Can you work these out from the model? Positions are in its coordinate system, mm. A direction names the side the tool comes from. Coordinates: 2 decimals unless noted, no trailing zeros. Loops run counter-clockwise (first coordinate to the right, second up) from the corner with the lowest first, then second, coordinate; pieces in that order, holes last.
```python
from build123d import *

# Parameters (mm, degrees)
SKETCH001_R                          = 4
SKETCH001_R_2                        = 1.4
SKETCH001_R_3                        = 2.75
EXTRUDE001_DEPTH                     = 20
SKETCH002_AS_DRAWN_W                 = 15
SKETCH002_AS_DRAWN_H                 = 13
SKETCH002_AS_DRAWN_R                 = 3.35
EXTRUDE002_DEPTH                     = 3
EXTRUDE002_ONTO_SKETCH002_ROLL_ANGLE = 90
SKETCH_R                             = 1.9
SKETCH_R_2                           = 23
SKETCH_R_3                           = 1.85
EXTRUDE_DEPTH                        = 3
CHAMFER_SIZE                         = 0.6


with BuildPart() as extrude001:
    # Sketch001 → Extrude001 (new body)
    with BuildSketch(Plane.XY):
        with Locations((-50.25, -47.25)):
            Circle(SKETCH001_R)
        with Locations((-50.25, -47.25)):
            Circle(SKETCH001_R_2, mode=Mode.SUBTRACT)
        with Locations((50.25, 47.25)):
            Circle(SKETCH001_R)
        with Locations((50.25, 47.25)):
            Circle(SKETCH001_R_2, mode=Mode.SUBTRACT)
        with Locations((-50.25, 47.25)):
            Circle(SKETCH001_R)
        with Locations((-50.25, 47.25)):
            Circle(SKETCH001_R_2, mode=Mode.SUBTRACT)
        with Locations((25.25, -42.25)):
            Circle(SKETCH001_R)
        with Locations((25.25, -42.25)):
            Circle(SKETCH001_R_2, mode=Mode.SUBTRACT)
        with Locations((51.25, -51.75)):
            Circle(SKETCH001_R_3)
        with Locations((-14.75, -39.25)):
            Circle(SKETCH001_R)
        with Locations((-14.75, -39.25)):
            Circle(SKETCH001_R_2, mode=Mode.SUBTRACT)
    extrude(amount=EXTRUDE001_DEPTH)


with BuildPart() as extrude002:
    # Sketch002 as drawn → Extrude002 (new)
    with BuildSketch(Plane.XY):
        with Locations((0, 6.5)):
            Rectangle(SKETCH002_AS_DRAWN_W, SKETCH002_AS_DRAWN_H)
        with Locations((0, 7)):
            Circle(SKETCH002_AS_DRAWN_R, mode=Mode.SUBTRACT)
    extrude(amount=-EXTRUDE002_DEPTH)


with BuildPart() as extrude002_1:
    # Extrude002 onto Sketch002 roll: moved
    add(extrude002.part.rotate(Axis((0, 0, 0), (1, 0, 0)), EXTRUDE002_ONTO_SKETCH002_ROLL_ANGLE))


with BuildPart() as extrude002_2:
    # Extrude002 onto Sketch002 placement: moved
    add(extrude002_1.part)


with BuildPart() as extrude002_3:
    # Extrude002 placement: moved
    add(extrude002_2.part.moved(Location((32, 61, 2))))


with BuildPart() as chamfer_body:
    # Sketch → Extrude (new body)
    with BuildSketch(Plane.XY):
        Polygon((55.5, 55), (55.5, -55), (-55.5, -55), (-55.5, 55), (24.5, 55), (24.5, 65), (39.5, 65), (39.5, 55), align=None)
        with Locations((-50.25, -47.25)):
            Circle(SKETCH_R, mode=Mode.SUBTRACT)
        Circle(SKETCH_R_2, mode=Mode.SUBTRACT)
        with Locations((-39.25, 47.25)):
            Circle(SKETCH_R_3, mode=Mode.SUBTRACT)
        with Locations((0.75, 47.25)):
            Circle(SKETCH_R_3, mode=Mode.SUBTRACT)
        with Locations((-39.25, 32.25)):
            Circle(SKETCH_R_3, mode=Mode.SUBTRACT)
        with Locations((0.75, 32.25)):
            Circle(SKETCH_R_3, mode=Mode.SUBTRACT)
        with Locations((10.75, 44.25)):
            Circle(SKETCH_R_3, mode=Mode.SUBTRACT)
        with Locations((40.75, 44.25)):
            Circle(SKETCH_R_3, mode=Mode.SUBTRACT)
        with Locations((10.75, 32.25)):
            Circle(SKETCH_R_3, mode=Mode.SUBTRACT)
        with Locations((40.75, 32.25)):
            Circle(SKETCH_R_3, mode=Mode.SUBTRACT)
        with Locations((50.25, 47.25)):
            Circle(SKETCH_R, mode=Mode.SUBTRACT)
        with Locations((-50.25, 47.25)):
            Circle(SKETCH_R, mode=Mode.SUBTRACT)
        with Locations((25.25, -42.25)):
            Circle(SKETCH_R, mode=Mode.SUBTRACT)
        with Locations((-14.75, -39.25)):
            Circle(SKETCH_R, mode=Mode.SUBTRACT)
        with Locations((-37.25, -7.25)):
            Circle(SKETCH_R_3, mode=Mode.SUBTRACT)
        with Locations((-37.25, -47.25)):
            Circle(SKETCH_R_3, mode=Mode.SUBTRACT)
    extrude(amount=EXTRUDE_DEPTH)

    # Fusion: union Extrude001, Extrude002
    add(extrude001.part)
    add(extrude002_3.part)

    # Chamfer
    chamfer_edges = [chamfer_body.edges().sort_by_distance(p)[0] for p in [
        (32, 61, 3),
        (32, 64, 3),
        (-54.25, -47.25, 3),
        (-18.75, -39.25, 3),
        (21.25, -42.25, 3),
        (-54.25, 47.25, 3),
        (46.25, 47.25, 3),
    ]]
    chamfer(chamfer_edges, length=CHAMFER_SIZE)


solid = chamfer_body.part
```
(1) If I drill on probe 1 along Y at (x, z) = (-37.25, 2.25); probe 2 along Y at (x, z) = (-50.25, 9.25); probe 3 along Y at (x, z) = (25.25, 7.25), over which ranges is the centre line in solid material (lowest first)?
Check values:
probe 1: y = -55 to -49.1, -45.4 to -9.1, -5.4 to 55
probe 2: y = -51.25 to -48.65, -45.85 to -43.25, 43.25 to 45.85, 48.65 to 51.25
probe 3: y = -46.25 to -43.65, -40.85 to -38.25, 61 to 64
(2) I want a section at B-B on y = 0. Write out the boundary of the cut face in (x, z), then the cut area to 3 significant figures.
Check values:
outline: (-55.5, 0) - (-23, 0) - (-23, 3) - (-55.5, 3) - close; (23, 0) - (55.5, 0) - (55.5, 3) - (23, 3) - close
area: 195 mm2
(3) If we mould it in two halves opening along Y, with no side actions, what happens to faces 1 (the cylindrical face through (-15.271, -35.284, 11.685)), 2 (the flat face through (50.2, 45.5, 20)), 3 (the cylindrical face through (-38.7, -48.4, 1.5))? For each: released by +Y, released by -Y, zero draft, split by the parting line, or undercut.
Check values:
face 1: split by the parting line
face 2: zero draft
face 3: undercut
(4) Which directions (+Z, -Z, +X, -X, +Y, -Y) give clear straight access to the entire face, cutting with the end or side of a thin tool? Please do faces 4 (the cylindrical face through (-54.246, -47.074, 11.685)), 5 (the flat face through (47, 55, 1)), 6 (the cylindrical face through (-40.614, 33.5, 1.479)).
Check values:
face 4: +Z
face 5: +Z, -Z, +X, +Y
face 6: +Z, -Z
(5) I want a section at D-D on y = -12.5. Write out the boundary of the cut face in (x, z).
Check values:
outline: (-55.5, 0) - (-19.31, 0) - (-19.31, 3) - (-55.5, 3) - close; (19.31, 0) - (55.5, 0) - (55.5, 3) - (19.31, 3) - close
(6) I want a section at A-A on z = 16.75. State how many separate pieces and enclosed holes the cut face has, then the cut area to 3 significant figures.
Check values:
separate pieces: 6
enclosed holes: 5
area: 244 mm2
(7) I'm going to push flat-ended pins straight in: pin 1 (11 mm diameter, centred on y = 62, z = 10.5, fed in from -X); pin 2 (8 mm diameter, centred on y = 52, z = 7.5, fed in from +X); pin 3 (0.9 mm diameter, centred on x = -32.5, z = 1.5, fed in from +Y); pin 4 (3 mm diameter, centred on x = -39.25, y = 32.25, fed in from +Z). Where does each tip first touch, or does it pass through?
Check values:
pin 1: stops at x = 24.5
pin 2: stops at x = 54.18
pin 3: stops at y = 55
pin 4: passes through
(8) I want a section at C-C on x = 34. Write out the boundary of the cut face in (y, z), then the cut area to 3 significant figures.
Check values:
outline: (-55, 0) - (65, 0) - (65, 3) - (64.6, 3) - (64, 3.6) - (64, 6.31) - (61, 6.31) - (61, 3.6) - (60.4, 3) - (-55, 3) - close; (61, 11.69) - (64, 11.69) - (64, 15) - (61, 15) - close
area: 380 mm2
